```python
from build123d import *

# Parameters (mm, degrees)
SKETCH_1_W      = 65
SKETCH_1_H      = 69.282032302
EXTRUDE_1_DEPTH = 65
FILLET_2_R      = 3


with BuildPart() as part:
    # Эскиз1 → Бобышка-Вытянуть1 (new body)
    with BuildSketch(Plane.XY):
        with BuildLine():
            Line((-32.5, 34.641016151), (32.5, 34.641016151))
            ThreePointArc((32.5, 34.641016151), (0, 47.5), (-32.5, 34.641016151))
        make_face()
        Rectangle(SKETCH_1_W, SKETCH_1_H)
        with BuildLine():
            ThreePointArc((-32.5, -34.641016151), (0, -47.5), (32.5, -34.641016151))
            Line((32.5, -34.641016151), (-32.5, -34.641016151))
        make_face()
    extrude(amount=EXTRUDE_1_DEPTH)

    # Скругление2
    fillet_2_edges = [part.edges().sort_by_distance(p)[0] for p in [
        (32.5, 34.641016151, 32.5),
        (32.5, -34.641016151, 32.5),
        (-32.5, -34.641016151, 32.5),
        (-32.5, 34.641016151, 32.5),
    ]]
    fillet(fillet_2_edges, radius=FILLET_2_R)


solid = part.part
```
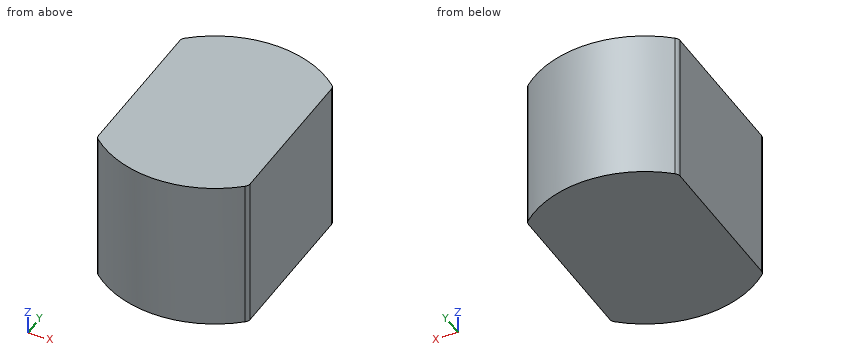
Check sheet for the modelled part. Datum: model origin and axes. Units: mm. Round coordinates to 2 decimals unless told otherwise and drop trailing zeros. Write each loop counter-clockwise with the first axis right and the second up, starting at its lowest first coordinate (ties: lowest second). Pieces come first, ordered by that corner, then holes. Notation, with made-up numbers: (19, 81.5) -> (49, 81.5) arc R17 ccw to (49, 93.5) -> close; hole circle Ø1 at (-16.75, 82). An arc over 180 degrees is marked (long way). Put each result on its own line as item: value.
(1) Sectioned sample at A-A (z = 23). Enter the section's corners in (x, y).
Values found:
outline: (-32.5, -33.32) arc R3 ccw to (-31.49, -35.56) arc R47.5 ccw to (31.49, -35.56) arc R3 ccw to (32.5, -33.32) -> (32.5, 33.32) arc R3 ccw to (31.49, 35.56) arc R47.5 ccw to (-31.49, 35.56) arc R3 ccw to (-32.5, 33.32) -> close
(2) Material ranges on line 1 (Y direction, x = 0, z = 24); line 2 (Y direction, x = 22.5, z = 46.5); line 3 (X direction, y = 34, z = 40), recorded low to high.
Values found:
line 1: y = -47.5 to 47.5
line 2: y = -41.83 to 41.83
line 3: x = -32.42 to 32.42
(3) Sectioned sample at C-C (x = 13). Enter the section's corners in (y, z), plus the area to 3 significant figures.
Values found:
outline: (-45.69, 0) -> (45.69, 0) -> (45.69, 65) -> (-45.69, 65) -> close
area: 5,940 mm^2
(4) Sectioned sample at B-B (y = 40). Enter the section's corners in (x, z).
Values found:
outline: (-25.62, 0) -> (25.62, 0) -> (25.62, 65) -> (-25.62, 65) -> close
(5) Go/stop test with flat-tipped pins: pin 1 Ø1.5 at (x, z) = (-0.5, 38.5) entering from +Y; pin 2 Ø2 at (x, z) = (-9, 50.5) entering from -Y; pin 3 Ø1 at (x, z) = (-19.5, 47.5) entering from +Y. Record where each tip stops, or that it passes through.
Values found:
pin 1: stops at y = 47.5
pin 2: stops at y = -46.82
pin 3: stops at y = 43.53
